Input: part model. Units: mm. Frame: model coordinates. Face numbers are marked on the shaded views. A direction names the side the tool comes from. Coordinates: 2 decimals unless noted, no trailing zeros. Loops run counter-clockwise (first coordinate to the right, second up) from the corner with the lowest first, then second, coordinate; pieces in that order, holes last.
(1) Line query: L1, parallel to X at y = -21, z = -23; L2, parallel to Y at x = -19, z = -18; L3, parallel to Y at x = -6.5, z = -17. Output: solid intervals per line, ascending.
(2) Section D-D, the plane x = 24. Return loops of the section in (y, z).
(3) Section C-C, the plane y = 2. Return loops of the section in (x, z).
(4) Mould query, pull axis Z, two halves, no side actions, for the marked faces 1, 2, 3 and 4. Classes: released by +Z, released by -Z, zero draft, split by the parting line, or undercut.
(5) Set-up query: the marked faces 5, 6, 7 and 8. Return all of +Z, -Z, +X, -X, +Y, -Y with unobstructed straight access to the full face (end or side cutting, diameter ignored); none if empty.
(6) Section A-A, the plane z = 3.5. Return loops of the section in (x, y), then the cut area to 3 significant figures.
(7) Contact query for flat-ended pins moving along their axis: P1, Ø8, axis at x = -9.5, z = -10, coming from the -Y side; P2, Ø1.8, axis at x = -8, z = -8, coming from the -Y side; P3, Ø10, axis at x = -14, y = -4.5, coming from the +Z side; P4, Ø6, axis at x = -3.5, y = 4.5, coming from the -Z side. Output: stop coordinate, or through.
```python
from build123d import *

# Parameters (mm, degrees)
F0_W      = 67
F0_H      = 55
F1_DEPTH  = 32.5
F3_DEPTH  = 33.5
F5_DEPTH  = 4.5
F8_DEPTH  = 6
F9_DEPTH  = 7
F11_D     = 5
F11_DEPTH = 13
F11_TIP   = 1.5021515476
F13_DEPTH = 18
F14_SIZE  = 6


with BuildPart() as f1:
    # F0 (on Front) → F1 (new body, symmetric)
    with BuildSketch(Plane.XZ):
        Rectangle(F0_W, F0_H)
    extrude(amount=F1_DEPTH, both=True)

    # F2 (on Right) → F3 (cut, symmetric)
    with BuildSketch(Plane.YZ):
        Polygon((-10, 4.5), (0, 4.5), (0, 27.5), (-15, 27.5), (-15, 17.5), (-20, 17.5), (-20, 9.5), (-10, 9.5), align=None)
        Polygon((0, 27.5), (0, 4.5), (10, 4.5), (10, 9.5), (20, 9.5), (20, 17.5), (15, 17.5), (15, 27.5), align=None)
        Polygon((10, -4.5), (0, -4.5), (0, -27.5), (15, -27.5), (15, -10.5), (10, -10.5), align=None)
        Polygon((0, -27.5), (0, -4.5), (-10, -4.5), (-10, -10.5), (-15, -10.5), (-15, -27.5), align=None)
    extrude(amount=F3_DEPTH, both=True, mode=Mode.SUBTRACT)

    # F4 (on Top) → F5 (cut, symmetric)
    with BuildSketch(Plane.XY):
        with BuildLine():
            ThreePointArc((20, 0), (18.8284271247, 2.8284271247), (16, 4))
            Line((16, 4), (-16, 4))
            ThreePointArc((-16, 4), (-18.8284271247, 2.8284271247), (-20, 0))
            ThreePointArc((-20, 0), (-18.8284271247, -2.8284271247), (-16, -4))
            Line((-16, -4), (16, -4))
            ThreePointArc((16, -4), (18.8284271247, -2.8284271247), (20, 0))
        make_face()
    extrude(amount=F5_DEPTH, both=True, mode=Mode.SUBTRACT)

    # F7 (on face) → F8 (cut)
    with BuildSketch(Plane(origin=(0, 32.5, 0), x_dir=(-1, 0, 0), z_dir=(0, 1, 0))):
        with BuildLine():
            Line((0, -3.5), (-3.5, -3.5))
            ThreePointArc((-3.5, -3.5), (-7.0355339059, -4.9644660941), (-8.5, -8.5))
            ThreePointArc((-8.5, -8.5), (-7.0355339059, -12.0355339059), (-3.5, -13.5))
            Line((-3.5, -13.5), (11.5, -13.5))
            ThreePointArc((11.5, -13.5), (15.0355339059, -12.0355339059), (16.5, -8.5))
            ThreePointArc((16.5, -8.5), (15.0355339059, -4.9644660941), (11.5, -3.5))
            Line((11.5, -3.5), (0, -3.5))
        make_face()
    extrude(amount=-F8_DEPTH, mode=Mode.SUBTRACT)

    # F6 (on face) → F9 (cut)
    with BuildSketch(Plane.XZ.offset(32.5)):
        with BuildLine():
            Line((0, -3.5220243782), (-11.4281616919, -3.5220243782))
            ThreePointArc((-11.4281616919, -3.5220243782), (-14.9636955978, -4.9864904722), (-16.4281616919, -8.5220243782))
            ThreePointArc((-16.4281616919, -8.5220243782), (-14.9636955978, -12.0575582841), (-11.4281616919, -13.5220243782))
            Line((-11.4281616919, -13.5220243782), (3.5718383081, -13.5220243782))
            ThreePointArc((3.5718383081, -13.5220243782), (7.1073722141, -12.0575582841), (8.5718383081, -8.5220243782))
            ThreePointArc((8.5718383081, -8.5220243782), (7.1073722141, -4.9864904722), (3.5718383081, -3.5220243782))
            Line((3.5718383081, -3.5220243782), (0, -3.5220243782))
        make_face()
    extrude(amount=-F9_DEPTH, mode=Mode.SUBTRACT)

    # F11
    with Locations(Plane(origin=(0, 0, -27.5), x_dir=(1, 0, 0), z_dir=(0, 0, -1))):
        with Locations((-19, -21), (-19, 21), (19, 21), (19, -21)):
            Hole(F11_D / 2, depth=F11_DEPTH)
            with Locations((0, 0, -(F11_DEPTH + F11_TIP / 2))):  # 118° drill point
                Cone(0, F11_D / 2, F11_TIP, mode=Mode.SUBTRACT)

    # F12 (on face) → F13 (cut)
    with BuildSketch(Plane.XY.offset(27.5)):
        Polygon((-33.5, 15), (-26, 15), (-33.5, 22.5), align=None)
        Polygon((33.5, 22.5), (26, 15), (33.5, 15), align=None)
        Polygon((26, -15), (33.5, -22.5), (33.5, -15), align=None)
        Polygon((-33.5, -15), (-33.5, -22.5), (-26, -15), align=None)
    extrude(amount=-F13_DEPTH, mode=Mode.SUBTRACT)

    # F14
    f14_edges = [f1.edges().sort_by_distance(p)[0] for p in [
        (33.5, -27.5, 27.5),
        (0, -32.5, 27.5),
        (-33.5, -27.5, 27.5),
        (33.5, 27.5, 27.5),
        (0, 32.5, 27.5),
        (-33.5, 27.5, 27.5),
    ]]
    chamfer(f14_edges, length=F14_SIZE)


solid = f1.part
```
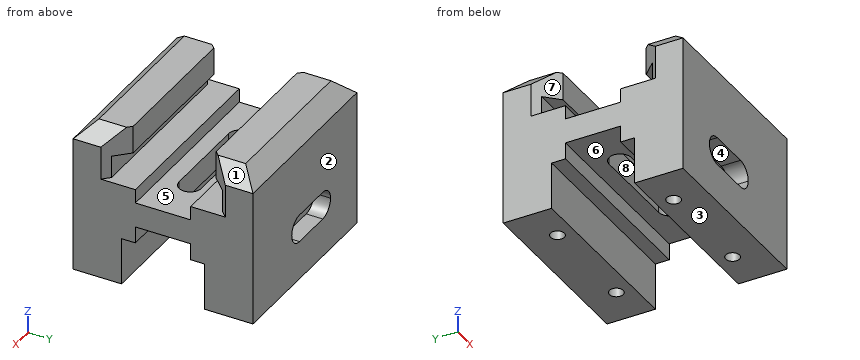
Report:
1. L1: x = -33.5 to -21.5, -16.5 to 16.5, 21.5 to 33.5
1. L2: y = -32.5 to -23.5, -18.5 to -15, 15 to 18.5, 23.5 to 32.5
1. L3: y = -32.5 to -15, 15 to 32.5
2. outline: (-32.5, -27.5) - (-15, -27.5) - (-15, -10.5) - (-10, -10.5) - (-10, -4.5) - (10, -4.5) - (10, -10.5) - (15, -10.5) - (15, -27.5) - (32.5, -27.5) - (32.5, 21.5) - (26.5, 27.5) - (15, 27.5) - (15, 17.5) - (20, 17.5) - (20, 9.5) - (10, 9.5) - (10, 4.5) - (-10, 4.5) - (-10, 9.5) - (-20, 9.5) - (-20, 17.5) - (-15, 17.5) - (-15, 27.5) - (-26.5, 27.5) - (-32.5, 21.5) - close
3. outline: (-33.5, -4.5) - (-19.46, -4.5) - (-19.46, 4.5) - (-33.5, 4.5) - close; (19.46, -4.5) - (33.5, -4.5) - (33.5, 4.5) - (19.46, 4.5) - close
4. face 1: released by +Z
4. face 2: zero draft
4. face 3: released by -Z
4. face 4: undercut
5. face 5: +Z, +X, -X
5. face 6: -Z, +X, -X
5. face 7: +Z, -X
5. face 8: +Z, -Z
6. outline: (-33.5, -32.5) - (33.5, -32.5) - (33.5, 32.5) - (-33.5, 32.5) - close; hole (-16, -4) - (16, -4) arc R4 ccw to (16, 4) - (-16, 4) arc R4 ccw to start
6. area: 4,050 mm2
7. P1: stops at y = -32.5
7. P2: stops at y = -25.5
7. P3: stops at z = 4.5
7. P4: stops at z = -4.5
